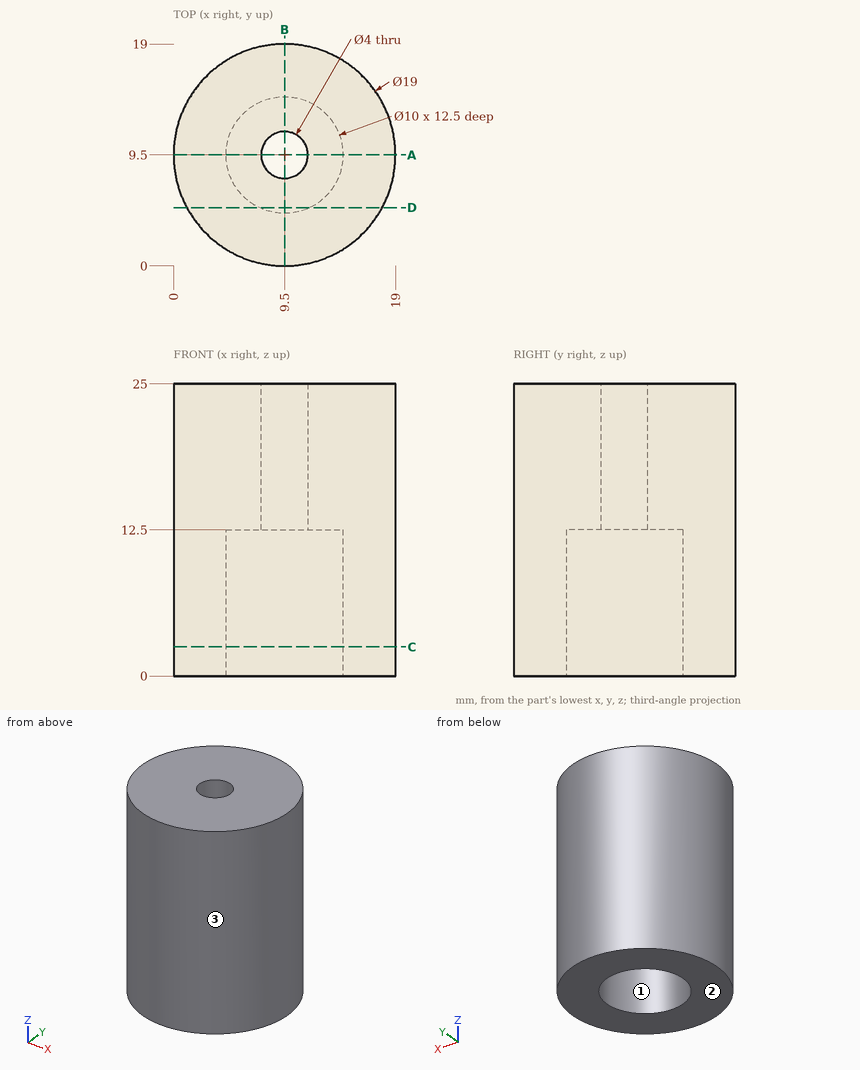
Geometry check sheet. Reference: drawing and pictorial views, mm from the part's lowest x, y, z. Round coordinates to 2 decimals unless told otherwise and drop trailing zeros. Order: outer loops, then holes, each group sorted by start corner. A loop starts at its lowest first (then second) coordinate and runs counter-clockwise, first axis right, second up. Notation, with made-up numbers: (71.25, -11.5) -> (81.25, -11.5) arc R21 cw to (81.25, 7.5) -> close; hole circle Ø4 at (21.5, 24). An arc over 180 degrees is marked (long way). One line per item, written item: value. Start each with the question number.
Q1. Gauge pin test, flat ends, axial feed: pin 1 Ø4 at (y, z) = (4.5, 16) entering from -X; pin 2 Ø5 at (x, z) = (6, 22) entering from -Y; pin 3 Ø8 at (x, z) = (3, 4.5) entering from +Y; pin 4 Ø3 at (x, y) = (9.5, 9.5) entering from -Z. Record the tip position at first contact, or that the pin passes through.
Q2. Cross-section at A-A (y = 9.5). Record the boundary of the cut face in (x, z).
Q3. Mould release check, pull along X, two halves, no side actions. Record for the marked faces 1, 2 and 3: pulls with the +X half, pulls with the -X half, needs draft (parallel to the pull), parting line crosses it, or undercut.
Q4. Thickness scan on line 1 (Y direction, x = 9.5, z = 4.25); line 2 (X direction, y = 13.5, z = 6.75); line 3 (X direction, y = 10.5, z = 19.5). Record the ranges inside material, lowest first.
Q5. Cross-section at C-C (z = 2.5). Record the boundary of the cut face in (x, y).
Q6. Cross-section at D-D (y = 5). Record the boundary of the cut face in (x, z), and give its area (3 significant figures).
Completed:
1. pin 1: stops at x = 0.49
1. pin 2: stops at y = 0.05
1. pin 3: stops at y = 18.67
1. pin 4: passes through
2. outline: (0, 0) -> (4.5, 0) -> (4.5, 12.5) -> (7.5, 12.5) -> (7.5, 25) -> (0, 25) -> close; (11.5, 12.5) -> (14.5, 12.5) -> (14.5, 0) -> (19, 0) -> (19, 25) -> (11.5, 25) -> close
3. face 1: undercut
3. face 2: needs draft
3. face 3: parting line crosses it
4. line 1: y = 0 to 4.5, 14.5 to 19
4. line 2: x = 0.88 to 6.5, 12.5 to 18.12
4. line 3: x = 0.05 to 7.77, 11.23 to 18.95
5. outline: circle Ø19 at (9.5, 9.5); hole circle Ø10 at (9.5, 9.5)
6. outline: (1.13, 0) -> (7.32, 0) -> (7.32, 12.5) -> (11.68, 12.5) -> (11.68, 0) -> (17.87, 0) -> (17.87, 25) -> (1.13, 25) -> close
6. area: 364 mm²
